Source: three-view drawing plus pictorial views. Frame: mm from the lowest corner of the part. A direction names the side the tool comes from. Round coordinates to 2 decimals unless told otherwise and drop trailing zeros. Loops run counter-clockwise (first coordinate to the right, second up) from the corner with the lowest first, then second, coordinate; pieces in that order, holes last. Notation, with made-up numbers: (45.5, 52.25) -> (56.5, 52.25) arc R26 ccw to (56.5, 71.25) -> close; hole circle Ø11 at (9, 47). An arc over 180 degrees is marked (long way). One line per question, with ' | ' between items. Start each with the question number.
Q1. Cut plane B-B on z = 55.5. Return loops of the section in (x, y), and give its area (3 significant figures).
Q2. Contact query for flat-ended pins moving along their axis: P1, Ø6, axis at y = 209.5, z = 49, coming from the -X side; P2, Ø10, axis at y = 188, z = 57.5, coming from the +X side; P3, Ø4, axis at x = 445.5, z = 97, coming from the -Y side (1 decimal). Output: stop coordinate, or through.
Q3. Material intervals for L1, parallel to X at y = 250, z = 9.5; L2, parallel to Y at x = 137.5, z = 119.5; L3, parallel to X at y = 318.5, z = 128, sorted ascending.
Q4. Cut plane C-C on x = 276.5. Return loops of the section in (y, z), and give its area (4 significant figures).
Q5. Cut plane D-D on z = 113.5. Return loops of the section in (x, y).
Q6. Access query for the marked faces 1, 2, 3 and 4. Directions: +Z, -Z, +X, -X, +Y, -Y. A direction counts if a zero-diameter tool reaches every point of the face in a straight line with its end or side. Return the directions, or none.
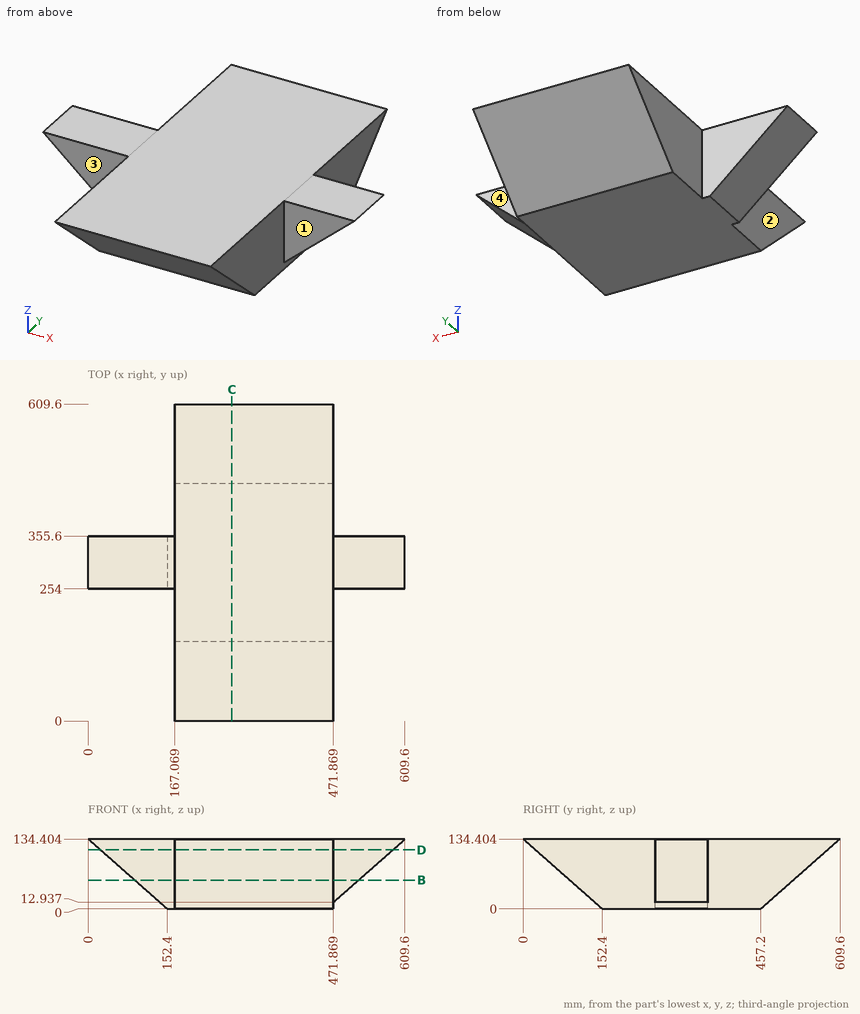
Results:
1) outline: (89.47, 254) -> (167.07, 254) -> (167.07, 89.47) -> (471.87, 89.47) -> (471.87, 254) -> (520.13, 254) -> (520.13, 355.6) -> (471.87, 355.6) -> (471.87, 520.13) -> (167.07, 520.13) -> (167.07, 355.6) -> (89.47, 355.6) -> close | area: 144,000 mm^2
2) P1: x = 167.07 | P2: x = 471.87 | P3: y = 40.1
3) L1: 167.07 to 471.87 | L2: 254 to 355.6 | L3: 7.26 to 602.34
4) outline: (0, 134.4) -> (152.4, 0) -> (457.2, 0) -> (609.6, 134.4) -> close | area: 61,450 mm^2
5) outline: (23.7, 254) -> (167.07, 254) -> (167.07, 23.7) -> (471.87, 23.7) -> (471.87, 254) -> (585.9, 254) -> (585.9, 355.6) -> (471.87, 355.6) -> (471.87, 585.9) -> (167.07, 585.9) -> (167.07, 355.6) -> (23.7, 355.6) -> close
6) face 1: +Z, -Z, +X, -Y | face 2: +Z, -Z, -X, -Y | face 3: +Z, -Z, -X, -Y | face 4: +Z, -Z, +X, +Y
